Could you check a few things on this drawing? It's one solid part, dimensions in mm from its lowest x, y, z. Give positions to 0.01 mm unless a question says otherwise; leave off trailing zeros. Loops run counter-clockwise (first coordinate to the right, second up) from the corner with the lowest first, then second, coordinate; pieces in that order, holes last. Notation, with made-up numbers: (16.25, 83.25) - (24.25, 83.25) arc R11 cw to (24.25, 97.25) - close; hole circle Ø1 at (86, -35). An arc over 180 degrees is marked (long way). Put each result on its own line as item: value. Start each with the question number.
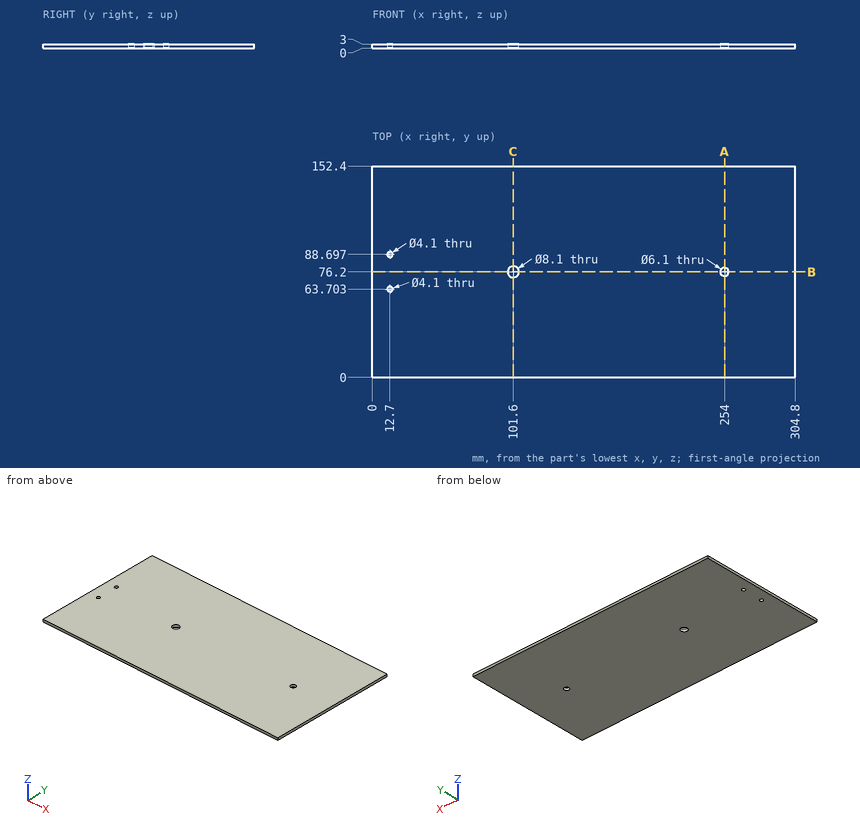
1) I need wall thicknesses on line 1 (Y direction, x = 12.7, z = 1.35); line 2 (X direction, y = 77, z = 1.3); line 3 (Y direction, x = 254, z = 1.85). Which ranges of each line are inside material? Lowest first, please.
2) Suppose I cut it at B-B on y = 76.2. Please give me the cut outline in (x, z).
3) I'm going to push a flat-ended pin straight in: P1, Ø3.5, axis at x = 12.7, y = 63.7, coming from the -Z side. Where does the tip first touch, or does it pass through?
4) Suppose I cut it at A-A on x = 254. Please give me the cut outline in (y, z).
5) Suppose I cut it at C-C on x = 101.6. Please give me the cut outline in (y, z), plus the area to 3 significant figures.
Ans:
1. line 1: y = 0 to 61.65, 65.75 to 86.65, 90.75 to 152.4
1. line 2: x = 0 to 97.63, 105.57 to 251.06, 256.94 to 304.8
1. line 3: y = 0 to 73.15, 79.25 to 152.4
2. outline: (0, 0) - (97.55, 0) - (97.55, 3) - (0, 3) - close; (105.65, 0) - (250.95, 0) - (250.95, 3) - (105.65, 3) - close; (257.05, 0) - (304.8, 0) - (304.8, 3) - (257.05, 3) - close
3. P1: passes through
4. outline: (0, 0) - (73.15, 0) - (73.15, 3) - (0, 3) - close; (79.25, 0) - (152.4, 0) - (152.4, 3) - (79.25, 3) - close
5. outline: (0, 0) - (72.15, 0) - (72.15, 3) - (0, 3) - close; (80.25, 0) - (152.4, 0) - (152.4, 3) - (80.25, 3) - close
5. area: 433 mm²
